```python
from build123d import *

# Parameters (mm, degrees)
SKETCH1_W           = 40
SKETCH1_H           = 30
BOSS_EXTRUDE1_DEPTH = 2.5
SKETCH2_R           = 5
BOSS_EXTRUDE2_DEPTH = 40
SKETCH4_R           = 2.25
CUT_EXTRUDE1_DEPTH  = 48.16990566


with BuildPart() as part:
    # Sketch1 → Boss-Extrude1 (new body)
    with BuildSketch(Plane(origin=(0, 0, 0), x_dir=(0, 0, -1), z_dir=(1, 0, 0))):
        Rectangle(SKETCH1_W, SKETCH1_H)
    extrude(amount=BOSS_EXTRUDE1_DEPTH)

    # Sketch2 → Boss-Extrude2 (add)
    with BuildSketch(Plane(origin=(2.5, 0, 0), x_dir=(0, 0, -1), z_dir=(1, 0, 0))):
        Circle(SKETCH2_R)
    extrude(amount=BOSS_EXTRUDE2_DEPTH)

    # Sketch4 → Cut-Extrude1 (cut, through all)
    with BuildSketch(Plane(origin=(2.5, 0, 0), x_dir=(0, 0, -1), z_dir=(1, 0, 0))):
        with Locations((-10, 10)):
            Circle(SKETCH4_R)
        with Locations((-10, -10)):
            Circle(SKETCH4_R)
        with Locations((10, 10)):
            Circle(SKETCH4_R)
        with Locations((10, -10)):
            Circle(SKETCH4_R)
    extrude(amount=-CUT_EXTRUDE1_DEPTH, mode=Mode.SUBTRACT)


solid = part.part
```
Geometry check sheet. Reference: the model listing, model coordinates, mm. A direction names the side the tool comes from. Coordinates: 2 decimals unless noted, no trailing zeros. Order: outer loops, then holes, each group sorted by start corner. A loop starts at its lowest first (then second) coordinate and runs counter-clockwise, first axis right, second up. Notation, with made-up numbers: (-7, -23) - (19, -23) arc R32 cw to (19, 4) - close; hole circle Ø2 at (12, 66.5). An arc over 180 degrees is marked (long way). Answer as a JSON object with one key per item and string values. Group by question number.
Item 1: Sectioned sample at A-A, the plane z = 10. Record the cut outline in (x, y), and give its area (3 significant figures).
Item 2: Scan lines: probe 1 along Y at (x, z) = (1.9, -10); probe 2 along X at (y, z) = (-4.25, -3.5); probe 3 along Z at (x, y) = (33.5, -3.5). Record each from-to range of solid material in increasing order.
Item 3: Draft check along Y on faces 1 (the face through (1, -15, 0)), 2 (the face through (1.27, 11.52, -8.34)), 3 (the face through (1.27, 11.52, 11.66)), 4 (the face through (1, 15, 0)). Enter one of: +Y half, -Y half, draft (parallel to the pull), parting line (faces both ways), or undercut.
Item 4: Tool access check on faces 5 (the face through (1, 0, 20)), 6 (the face through (22.22, -4.88, 1.08)). Record the directions out of +Z, -Z, +X, -X, +Y, -Y that give a thin tool (end or side, any length) a straight path to the whole face; none if there is none.
Item 5: Sectioned sample at D-D, the plane y = 2. Record the cut outline in (x, z), and give its area (3 significant figures).
Item 6: Sectioned sample at B-B, the plane y = -10. Record the cut outline in (x, z).
Item 7: Depth check by flat-ended pin: pin 1 Ø8 at (x, z) = (34.5, -12) entering from +Y; pin 2 Ø3 at (x, y) = (28, 3) entering from -Z; pin 3 Ø4 at (x, z) = (19.5, -4) entering from -Y; pin 4 Ø1 at (x, z) = (19, -0.5) entering from +Y. Enter the tip coordinate at first touch or a pass-through.
Item 8: Sectioned sample at C-C, the plane x = 7. Record the cut outline in (y, z).
Resolved:
{
 "1": {"outline": "(0, -15) - (2.5, -15) - (2.5, -12.25) - (0, -12.25) - close; (0, -7.75) - (2.5, -7.75) - (2.5, 7.75) - (0, 7.75) - close; (0, 12.25) - (2.5, 12.25) - (2.5, 15) - (0, 15) - close", "area": "52.5 mm^2"},
 "2": {"probe 1": "-15 to -12.25, -7.75 to 7.75, 12.25 to 15", "probe 2": "0 to 2.5", "probe 3": "-3.57 to 3.57"},
 "3": {"face 1": "-Y half", "face 2": "undercut", "face 3": "undercut", "face 4": "+Y half"},
 "4": {"face 5": "+Z, +X, -X, +Y, -Y", "face 6": "+X"},
 "5": {"outline": "(0, -20) - (2.5, -20) - (2.5, -4.58) - (42.5, -4.58) - (42.5, 4.58) - (2.5, 4.58) - (2.5, 20) - (0, 20) - close", "area": "467 mm^2"},
 "6": {"outline": "(0, -20) - (2.5, -20) - (2.5, -12.25) - (0, -12.25) - close; (0, -7.75) - (2.5, -7.75) - (2.5, 7.75) - (0, 7.75) - close; (0, 12.25) - (2.5, 12.25) - (2.5, 20) - (0, 20) - close"},
 "7": {"pin 1": "through", "pin 2": "z = -4.77", "pin 3": "y = -4.58", "pin 4": "y = 5"},
 "8": {"outline": "circle Ø10 at (0, 0)"}
}
